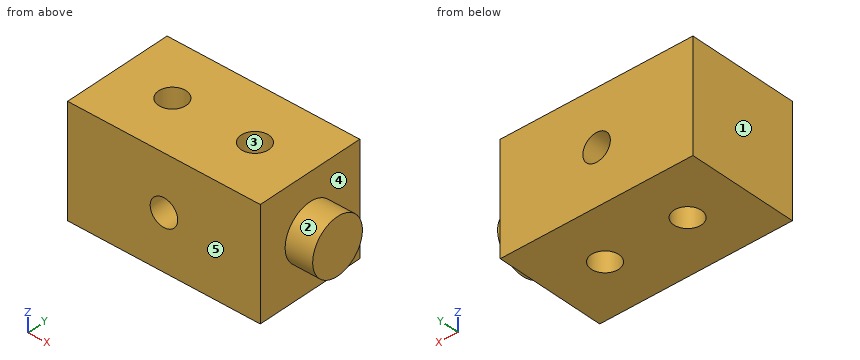
```python
from build123d import *

# Parameters (mm, degrees)
SKETCH1_W           = 44.45
SKETCH1_H           = 25.4
SKETCH1_R           = 3.175
BOSS_EXTRUDE1_DEPTH = 25.4
SKETCH2_R           = 6.35
BOSS_EXTRUDE2_DEPTH = 6.35
SKETCH3_R           = 3.175
CUT_EXTRUDE1_DEPTH  = 63.217039467


with BuildPart() as part:
    # Sketch1 → Boss-Extrude1 (new body)
    with BuildSketch(Plane.XY):
        with Locations((22.225, 12.7)):
            Rectangle(SKETCH1_W, SKETCH1_H)
        with Locations((12.7, 12.7)):
            Circle(SKETCH1_R, mode=Mode.SUBTRACT)
        with Locations((31.75, 12.7)):
            Circle(SKETCH1_R, mode=Mode.SUBTRACT)
    extrude(amount=BOSS_EXTRUDE1_DEPTH)

    # Sketch2 → Boss-Extrude2 (add)
    with BuildSketch(Plane(origin=(44.45, 0, 0), x_dir=(0, 0, -1), z_dir=(1, 0, 0))):
        with Locations((-12.7, 12.7)):
            Circle(SKETCH2_R)
    extrude(amount=BOSS_EXTRUDE2_DEPTH)

    # Sketch3 → Cut-Extrude1 (cut, through all)
    with BuildSketch(Plane(origin=(0, 25.4, 0), x_dir=(1, 0, 0), z_dir=(0, 1, 0))):
        with Locations(Location((22.225, -12.7, 0), (0, 0, 270))):
            Circle(SKETCH3_R)
    extrude(amount=-CUT_EXTRUDE1_DEPTH, mode=Mode.SUBTRACT)


solid = part.part
```
Could you check a few things on this model? Use its own coordinates, in mm. Face numbers are marked on the shaded views. A direction names the side the tool comes from. Give positions to 0.01 mm unless a question says otherwise; leave off trailing zeros. Loops run counter-clockwise (first coordinate to the right, second up) from the corner with the lowest first, then second, coordinate; pieces in that order, holes last. Notation, with made-up numbers: (58.5, -32) - (101.5, -32) arc R17 cw to (101.5, -23) - close; hole circle Ø11 at (-33, 11). An arc over 180 degrees is marked (long way). Use one line per item in the form item = value.
1. I need wall thicknesses on probe 1 along Y at (x, z) = (31.75, 11.75) (3 decimals); probe 2 along X at (y, z) = (15.25, 22.25); probe 3 along X at (y, z) = (16.5, 12.5). Which ranges of each line are inside material? Lowest first, please.
Response values:
probe_1 = 0 to 9.525, 15.875 to 25.4
probe_2 = 0 to 10.81, 14.59 to 29.86, 33.64 to 44.45
probe_3 = 0 to 19.06, 25.39 to 50.8
2. I want a section at A-A (z = 12.7). Please give me the cut outline in (x, y) (3 decimals), and give its area (3 significant figures).
Response values:
outline = (0, 0) - (19.05, 0) - (19.05, 25.4) - (0, 25.4) - close; (25.4, 0) - (44.45, 0) - (44.45, 6.35) - (50.8, 6.35) - (50.8, 19.05) - (44.45, 19.05) - (44.45, 25.4) - (25.4, 25.4) - close; hole circle Ø6.35 at (12.7, 12.7); hole circle Ø6.35 at (31.75, 12.7)
area = 985 mm²
3. Thinking about a two-plate mould opening in X: for the marked faces 1, 2 and 3, which applies, released by +X, released by -X, zero draft, split by the parting line, or undercut?
Response values:
face_1 = released by -X
face_2 = zero draft
face_3 = undercut
4. I want a section at B-B (x = 12.7). Please give me the cut outline in (y, z) (3 decimals), and give its area (3 significant figures).
Response values:
outline = (0, 0) - (9.525, 0) - (9.525, 25.4) - (0, 25.4) - close; (15.875, 0) - (25.4, 0) - (25.4, 25.4) - (15.875, 25.4) - close
area = 484 mm²
5. I want a section at D-D (z = 23.75). Please give me the cut outline in (x, y) (3 decimals).
Response values:
outline = (0, 0) - (44.45, 0) - (44.45, 25.4) - (0, 25.4) - close; hole circle Ø6.35 at (12.7, 12.7); hole circle Ø6.35 at (31.75, 12.7)
6. I want a section at C-C (y = 12.7). Please give me the cut outline in (x, z) (3 decimals).
Response values:
outline = (0, 0) - (9.525, 0) - (9.525, 25.4) - (0, 25.4) - close; (15.875, 0) - (28.575, 0) - (28.575, 25.4) - (15.875, 25.4) - close; (34.925, 0) - (44.45, 0) - (44.45, 6.35) - (50.8, 6.35) - (50.8, 19.05) - (44.45, 19.05) - (44.45, 25.4) - (34.925, 25.4) - close; hole circle Ø6.35 at (22.225, 12.7)
7. On a 3-axis mill with a long thin cutter (end or side, diameter ignored), from which of +Z, -Z, +X, -X, +Y, -Y can I reach the whole of each face in a straight line? I mean the marked faces 4 and 5. Say none if no direction works.
Response values:
face_4 = +X
face_5 = +Z, -Z, +X, -X, -Y
